CAD build for the part. Positions are in the model's coordinates, mm. Face numbers are marked on the shaded views. A direction names the side the tool comes from. Coordinates: 2 decimals unless noted, no trailing zeros. Order: outer loops, then holes, each group sorted by start corner. A loop starts at its lowest first (then second) coordinate and runs counter-clockwise, first axis right, second up. Notation, with made-up numbers: M 79,54.25 L 97,54.25 A20 cw 97,64.25 Z; hole C 55,76 d6. An arc over 180 degrees is marked long. Write item = value, one per line.
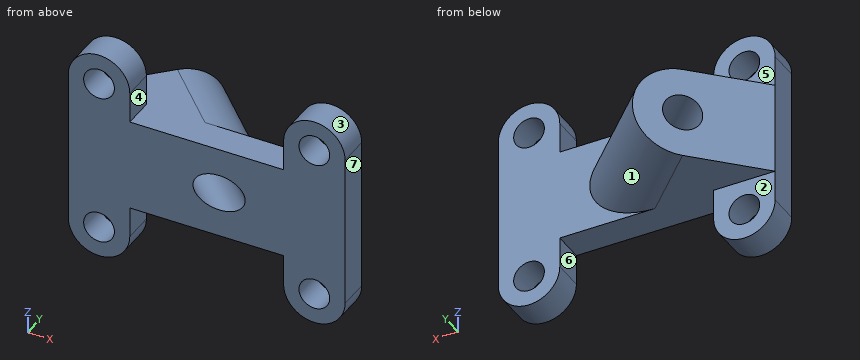
from build123d import *

# Parameters (mm, degrees)
SKETCH_1_R          = 2.5
EXTRUDE_1_DEPTH     = 5
EXTRUDE_3_REACH     = 37.355
SKETCH_6_R          = 3
SKETCH_9_R          = 3
CUT_EXTRUDE_2_DEPTH = 36.355339059


with BuildPart() as part:
    # 草圖1 → 填料-伸長1 (new body)
    with BuildSketch(Plane(origin=(0, 0, 0), x_dir=(1, 0, 0), z_dir=(0, 1, 0))):
        with BuildLine():
            Line((-12.5, 7.5), (12.5, 7.5))
            Line((12.5, 7.5), (12.5, 12.5))
            ThreePointArc((12.5, 12.5), (17.5, 17.5), (22.5, 12.5))
            Line((22.5, 12.5), (22.5, -12.5))
            ThreePointArc((22.5, -12.5), (17.5, -17.5), (12.5, -12.5))
            Line((12.5, -12.5), (12.5, -7.5))
            Line((12.5, -7.5), (-12.5, -7.5))
            Line((-12.5, -7.5), (-12.5, -12.5))
            ThreePointArc((-12.5, -12.5), (-17.5, -17.5), (-22.5, -12.5))
            Line((-22.5, -12.5), (-22.5, 12.5))
            ThreePointArc((-22.5, 12.5), (-17.5, 17.5), (-12.5, 12.5))
            Line((-12.5, 12.5), (-12.5, 7.5))
        make_face()
        with Locations((-17.5, -12.5)):
            Circle(SKETCH_1_R, mode=Mode.SUBTRACT)
        with Locations((-17.5, 12.5)):
            Circle(SKETCH_1_R, mode=Mode.SUBTRACT)
        with Locations((17.5, -12.5)):
            Circle(SKETCH_1_R, mode=Mode.SUBTRACT)
        with Locations((17.5, 12.5)):
            Circle(SKETCH_1_R, mode=Mode.SUBTRACT)
    extrude(amount=EXTRUDE_1_DEPTH)

    # 填料-伸長3: up to this face of the body (flat: up to its plane)
    extrude_3_end = Plane(part.part.faces().sort_by_distance((0, 0, 0))[0])
    # 草圖6 → 填料-伸長3 (add, up to the picked face)
    with BuildSketch(Plane(origin=(-13.75, 13.75, 0), x_dir=(0, 0, 1), z_dir=(-0.707106781, 0.707106781, 0)), mode=Mode.PRIVATE) as extrude_3_sk1:
        with BuildLine():
            Line((-7.5, -12.374368671), (-7.5, 1.425631329))
            ThreePointArc((-7.5, 1.425631329), (0, 8.925631329), (7.5, 1.425631329))
            Line((7.5, 1.425631329), (7.5, -12.374368671))
            Line((7.5, -12.374368671), (-7.5, -12.374368671))
        make_face()
        with Locations((0, 1.425631329)):
            Circle(SKETCH_6_R, mode=Mode.SUBTRACT)
    extrude_3_tool1 = split(extrude(extrude_3_sk1.sketch, amount=-EXTRUDE_3_REACH, mode=Mode.PRIVATE), bisect_by=extrude_3_end, keep=Keep.BOTH, mode=Mode.PRIVATE)
    add(extrude_3_tool1.solids().sort_by_distance((-15.778761, 11.721239, 0))[0])

    # 草圖9 → 除料-伸長2 (cut, through all)
    with BuildSketch(Plane(origin=(-13.75, 13.75, 0), x_dir=(0, 0, 1), z_dir=(-0.707106781, 0.707106781, 0))):
        with Locations((0, 1.425631329)):
            Circle(SKETCH_9_R)
    extrude(amount=-CUT_EXTRUDE_2_DEPTH, mode=Mode.SUBTRACT)


solid = part.part
(1) Slice it at C-C, the plane z = -13. Write the cut outline in (x, y).
Evaluation:
outline = M -22.47,0 L -19.95,0 L -19.95,5 L -22.47,5 Z; M -15.05,0 L -12.53,0 L -12.53,5 L -15.05,5 Z; M 12.53,0 L 15.05,0 L 15.05,5 L 12.53,5 Z; M 19.95,0 L 22.47,0 L 22.47,5 L 19.95,5 Z
(2) Tool access for the marked faces 5, 6 and 7: list every direction of +Z, -Z, +X, -X, +Y, -Y with a clear straight run to the whole face (end or side of a thin tool).
Evaluation:
face_5 = +Z, +X, -X, +Y
face_6 = -Z, +Y, -Y
face_7 = +Z, -Z, +X, +Y, -Y
(3) Pull direction X, two halves, no side cores. Call the marked faces 1, 2, 3 and 4: +X half, -X half, draft (parallel to the pull), parting line (faces both ways), or undercut.
Evaluation:
face_1 = +X half
face_2 = draft
face_3 = undercut
face_4 = undercut
(4) Slice it at A-A, the plane z = -9.5. Write the cut outline in (x, y), then the cut area to 3 significant figures.
Evaluation:
outline = M -22.5,0 L -12.5,0 L -12.5,5 L -22.5,5 Z; M 12.5,0 L 22.5,0 L 22.5,5 L 12.5,5 Z
area = 100 mm²
(5) Slice it at B-B, the plane x = -17.5. Write the cut outline in (y, z), then the cut area to 3 significant figures.
Evaluation:
outline = M 0,-17.5 L 5,-17.5 L 5,-15 L 0,-15 Z; M 0,-10 L 5,-10 L 5,-7.5 L 10,-7.5 L 10,7.5 L 5,7.5 L 5,10 L 0,10 Z; M 0,15 L 5,15 L 5,17.5 L 0,17.5 Z
area = 200 mm²
(6) Wall check: line 1 (Z direction, x = -17.5, y = 2.1); line 2 (X direction, y = 1.8, z = -12.5); line 3 (Z direction, x = 16, y = 3.5). Give the ranges that are in metal, low to high. Write a range as from..to.
Evaluation:
line_1 = -17.5..-15, -10..10, 15..17.5
line_2 = -22.5..-20, -15..-12.5, 12.5..15, 20..22.5
line_3 = -17.27..-14.5, -10.5..10.5, 14.5..17.27
(7) Pin check, flat tips, straight feed: pin 1 Ø7.5 at (x, z) = (4.5, 5.5) entering from +Y; pin 2 Ø5 at (x, z) = (-15.5, 10.5) entering from +Y; pin 3 Ø3 at (y, z) = (9.5, -6.5) entering from +X. Stop position of each tip, or through.
Evaluation:
pin_1 = 10.08
pin_2 = 5
pin_3 = 0.92
(8) Slice it at D-D, the plane x = 17.5. Write the cut outline in (y, z), then the cut area to 3 significant figures.
Evaluation:
outline = M 0,-17.5 L 5,-17.5 L 5,-15 L 0,-15 Z; M 0,-10 L 5,-10 L 5,10 L 0,10 Z; M 0,15 L 5,15 L 5,17.5 L 0,17.5 Z
area = 125 mm²
